Geometry: final body of the model. Coordinates: model frame, mm. A direction names the side the tool comes from. Round coordinates to 2 decimals unless told otherwise and drop trailing zeros. Write each loop counter-clockwise with the first axis right and the second up, starting at its lowest first coordinate (ties: lowest second). Pieces come first, ordered by that corner, then holes. Notation, with made-up numbers: M -4.5,86 L 19.5,86 A13 ccw 19.5,102 Z; hole C 1.5,54 d1. An arc over 180 degrees is marked long. Use one line per item in the form item = value. Start each with the question number.
from build123d import *

# Parameters (mm, degrees)
SKETCH_2_R      = 1.5
EXTRUDE_1_DEPTH = 2
EXTRUDE_2_DEPTH = 4
FILLET_1_R      = 1
FILLET_4_R      = 0.5


with BuildPart() as part:
    # 草图2 → 凸台-拉伸1 (new body)
    with BuildSketch(Plane.XY):
        with BuildLine():
            Line((7, 6), (-7, 6))
            Line((-7, 6), (-16, 6))
            Line((-16, 6), (-16, 0))
            ThreePointArc((-16, 0), (-14.108952351, -5.519311231), (-9.230489674, -8.71922679))
            Line((-9.230489674, -8.71922679), (-0.619580465, -10.922007442))
            ThreePointArc((-0.619580465, -10.922007442), (0, -11), (0.619580465, -10.922007442))
            Line((0.619580465, -10.922007442), (9.230489674, -8.71922679))
            ThreePointArc((9.230489674, -8.71922679), (14.108952351, -5.519311231), (16, 0))
            Line((16, 0), (16, 6))
            Line((16, 6), (7, 6))
        make_face()
        with Locations((0, -8.5)):
            Circle(SKETCH_2_R, mode=Mode.SUBTRACT)
        with Locations((7, 0)):
            Circle(SKETCH_2_R, mode=Mode.SUBTRACT)
        with Locations(Location((-7, 0, 0), (0, 0, 180))):
            Circle(SKETCH_2_R, mode=Mode.SUBTRACT)
    extrude(amount=EXTRUDE_1_DEPTH)

    # 草图3 → 凸台-拉伸2 (add)
    with BuildSketch(Plane.XY.offset(2)):
        with BuildLine():
            Line((13.5, 0), (16, 0))
            ThreePointArc((16, 0), (14.527522767, -4.933193793), (10.591910889, -8.252161909))
            Line((10.591910889, -8.252161909), (9.594157864, -5.959894712))
            ThreePointArc((9.594157864, -5.959894712), (12.43654422, -3.562862184), (13.5, 0))
        make_face()
    extrude(amount=EXTRUDE_2_DEPTH)

    # 圆角1
    fillet_1_edges = [part.edges().sort_by_distance(p)[0] for p in [
        (-16, 6, 1),
        (16, 6, 1),
    ]]
    fillet(fillet_1_edges, radius=FILLET_1_R)

    # 圆角4
    fillet_4_edges = [part.edges().sort_by_distance(p)[0] for p in [
        (10.591910889, -8.252161909, 4),
        (16, 0, 4),
        (13.5, 0, 4),
        (9.594157864, -5.959894712, 4),
    ]]
    fillet(fillet_4_edges, radius=FILLET_4_R)


solid = part.part
1. Ray query, probe 1 along Z at (x, y) = (-2.5, 4.5); probe 2 along Y at (x, z) = (-7, 0.5); probe 3 along X at (y, z) = (-8, 5.5). Return the intervals inside material, ascending.
2. Section query A-A (z = 0.5). Return loops of the section in (x, y), then the cut area to 3 significant figures.
3. Pull-direction query (X, two-part tool) for faces 4 (the face through (16, 2, 1)), 5 (the face through (0, -10, 1)), 6 (the face through (13, -4, 6)), 7 (the face through (12.41, -3.6, 3.97)); classes: released by +X, released by -X, zero draft, split by the parting line, or undercut.
4. Section query D-D (y = 2.5). Return loops of the section in (x, z), then the cut area to 3 significant figures.
5. Section query B-B (x = 0). Return loops of the section in (y, z).
6. Set-up query: faces 1 (the face through (15, 0, 4)), 2 (the face through (10.09, -7.1, 3.97)), 3 (the face through (0, -11, 1)). Return all of +Z, -Z, +X, -X, +Y, -Y with unobstructed straight access to the full face (end or side cutting, diameter ignored); none if empty.
7. Section query C-C (z = 4). Return loops of the section in (x, y).
8. Contact query for flat-ended pins moving along their axis: pin 1 (1 mm diameter, centred on y = -1.5, z = 5.5, fed in from +X); pin 2 (10 mm diameter, centred on x = 8.5, y = -4.5, fed in from +Z); pin 3 (4 mm diameter, centred on x = -7, y = 0, fed in from +Z); pin 4 (0.5 mm diameter, centred on x = 14.5, z = 5, fed in from +Y). Output: stop coordinate, or through.
Checks:
q1.probe_1 = 0 to 2
q1.probe_2 = -9.29 to -1.5, 1.5 to 6
q1.probe_3 = 10.57 to 11.12
q2.outline = M -16,0 A9 ccw -9.23,-8.72 L -0.62,-10.92 A2.5 ccw 0.62,-10.92 L 9.23,-8.72 A9 ccw 16,0 L 16,5 A1 ccw 15,6 L -15,6 A1 ccw -16,5 Z; hole C -7,0 d3; hole C 0,-8.5 d3; hole C 7,0 d3
q2.area = 441 mm^2
q3.face_4 = released by +X
q3.face_5 = undercut
q3.face_6 = zero draft
q3.face_7 = released by -X
q4.outline = M -16,0 L 16,0 L 16,2 L -16,2 Z
q4.area = 64.0 mm^2
q5.outline = M -11,0 L -10,0 L -10,2 L -11,2 Z; M -7,0 L 6,0 L 6,2 L -7,2 Z
q6.face_1 = +Z, +X, -X, +Y
q6.face_2 = +Z, -X, -Y
q6.face_3 = +Z, -Z, -Y
q7.outline = M 9.79,-6.4 L 10.39,-7.78 A0.5 ccw 11.07,-8.03 A9 ccw 15.98,-0.53 A0.5 ccw 15.49,0 L 13.98,0 A0.5 ccw 13.48,-0.46 A6.5 cw 10.01,-5.76 A0.5 ccw Z
q8.pin_1 = 15.94
q8.pin_2 = 6
q8.pin_3 = 2
q8.pin_4 = 0
